Source: CAD feature listing. Evaluate the final solid. Frame: model axes, mm. Face numbers are marked on the shaded views. Coordinates: 2 decimals unless noted, no trailing zeros. Loops run counter-clockwise (first coordinate to the right, second up) from the corner with the lowest first, then second, coordinate; pieces in that order, holes last. Notation, with made-up numbers: M 0.5,-19 L 17.5,-19 A27 cw 17.5,1 Z; hole C 73.25,42 d7. An arc over 180 degrees is marked long. One line per question, with ' | ' between items. Start each with the question number.
1. Section query C-C, the plane x = 4. Output: boundary loops of the cut face in (y, z).
2. Pin query (flat end, axial travel): P1, Ø3, axis at x = 12.5, y = 0.5, coming from the +Z side; P2, Ø3, axis at x = 0, y = 0, coming from the -Z side; P3, Ø4, axis at x = -32.5, y = 0, coming from the -Z side; P4, Ø3, axis at x = -25, z = -17.5, coming from the +Y side. Return the tip coordinate at first contact, or that it passes through.
3. Section query A-A, the plane x = 25. Output: boundary loops of the cut face in (y, z).
4. Ray query, probe 1 along X at (y, z) = (-0.25, -13); probe 2 along Z at (x, y) = (25, -0.5); probe 3 along X at (y, z) = (-0.5, -17.5). Return the intervals inside material, ascending.
5. Section query B-B, the plane z = -17.5. Output: boundary loops of the cut face in (x, y), and give its area (3 significant figures).
6. Mould query, pull axis Z, two halves, no side actions, for the marked faces 1 and 2. Classes: pulls with the +Z half, pulls with the -Z half, needs draft (parallel to the pull), parting line crosses it, or undercut.
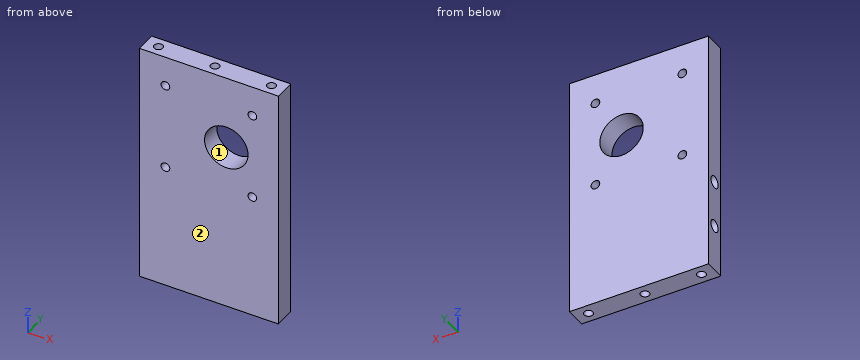
```python
from build123d import *

# Parameters (mm, degrees)
SKETCH1_W                  = 80
SKETCH1_H                  = 140
SKETCH1_R                  = 12.5
BOSS_EXTRUDE1_DEPTH        = 6
M6_TAPPED_HOLE1_D          = 5
M6_TAPPED_HOLE2_AT_2_COUNT = 2
M6_TAPPED_HOLE2_AT_2_PITCH = 32.5
M6_TAPPED_HOLE2_AT_3_COUNT = 2
M6_TAPPED_HOLE2_AT_3_PITCH = 65
M8X1_0_TAPPED_HOLE1_D      = 7
M8X1_0_TAPPED_HOLE1_DEPTH  = 19
M8X1_0_TAPPED_HOLE1_TIP    = 2.103012167


with BuildPart() as part:
    # Sketch1 → Boss-Extrude1 (new body, symmetric)
    with BuildSketch(Plane(origin=(0, 0, 0), x_dir=(1, 0, 0), z_dir=(0, 1, 0))):
        with Locations((0, 70)):
            Rectangle(SKETCH1_W, SKETCH1_H)
        with Locations((10, 42.5)):
            Circle(SKETCH1_R, mode=Mode.SUBTRACT)
    extrude(amount=BOSS_EXTRUDE1_DEPTH, both=True)

    # M6 Tapped Hole1 (through all)
    with Locations(Plane(origin=(0, 6, 0), x_dir=(1, 0, 0), z_dir=(0, 1, 0))):
        with Locations((-25, 67.5), (25, 67.5), (25, 17.5), (-25, 17.5)):
            Hole(M6_TAPPED_HOLE1_D / 2)

    # Sketch9 → M6 Tapped Hole2 (revolve, cut)
    with BuildSketch(Plane(origin=(32.5, 0, 0), x_dir=(0, -1, 0), z_dir=(1, 0, 0))):
        Polygon((0, 0), (0, 14.502151548), (2.5, 13), (2.5, 0), align=None)
    m6_tapped_hole2 = revolve(axis=Axis((32.5, 0, 6.35), (0, 0, -1)), mode=Mode.SUBTRACT)

    # M6 Tapped Hole2 at 2: M6 Tapped Hole2 ×2
    with Locations(*[(-i * M6_TAPPED_HOLE2_AT_2_PITCH, 0, 0) for i in range(1, M6_TAPPED_HOLE2_AT_2_COUNT)]):
        add(m6_tapped_hole2, mode=Mode.SUBTRACT)

    # M6 Tapped Hole2 at 3: M6 Tapped Hole2 ×2
    with Locations(*[(-i * M6_TAPPED_HOLE2_AT_3_PITCH, 0, 0) for i in range(1, M6_TAPPED_HOLE2_AT_3_COUNT)]):
        add(m6_tapped_hole2, mode=Mode.SUBTRACT)

    # Mirror1: M6 Tapped Hole2 across plane
    add(m6_tapped_hole2.mirror(Plane(origin=(0, 0, -70), x_dir=(1, 0, 0), z_dir=(0, 0, -1))), mode=Mode.SUBTRACT)

    # Mirror1 copy 1 sketch → Mirror1 copy 1 (revolve, cut)
    with BuildSketch(Plane(origin=(0, 0, -140), x_dir=(0, -1, 0), z_dir=(1, 0, 0))):
        Polygon((0, 0), (0, -14.502151548), (2.5, -13), (2.5, 0), align=None)
    revolve(axis=Axis((0, 0, -146.35), (0, 0, -1)), mode=Mode.SUBTRACT)

    # Mirror1 copy 2 sketch → Mirror1 copy 2 (revolve, cut)
    with BuildSketch(Plane(origin=(-32.5, 0, -140), x_dir=(0, -1, 0), z_dir=(1, 0, 0))):
        Polygon((0, 0), (0, -14.502151548), (2.5, -13), (2.5, 0), align=None)
    revolve(axis=Axis((-32.5, 0, -146.35), (0, 0, -1)), mode=Mode.SUBTRACT)

    # M8x1.0 Tapped Hole1
    with Locations(Plane.ZY.offset(40)):
        with Locations((-113, 0), (-86, 0)):
            Hole(M8X1_0_TAPPED_HOLE1_D / 2, depth=M8X1_0_TAPPED_HOLE1_DEPTH)
            with Locations((0, 0, -(M8X1_0_TAPPED_HOLE1_DEPTH + M8X1_0_TAPPED_HOLE1_TIP / 2))):  # 118° drill point
                Cone(0, M8X1_0_TAPPED_HOLE1_D / 2, M8X1_0_TAPPED_HOLE1_TIP, mode=Mode.SUBTRACT)


solid = part.part
```
Taken from the geometry:
1) outline: M -6,-140 L 6,-140 L 6,-53.47 L -6,-53.47 Z; M -6,-31.53 L 6,-31.53 L 6,0 L -6,0 Z
2) P1: z = 0 | P2: z = -126.4 | P3: z = -126.7 | P4: through
3) outline: M -6,-140 L 6,-140 L 6,-70 L -6,-70 Z; M -6,-65 L 6,-65 L 6,-20 L -6,-20 Z; M -6,-15 L 6,-15 L 6,0 L -6,0 Z
4) probe 1: -40 to -34.99, -30.01 to -2.49, 2.49 to 30.01, 34.99 to 40 | probe 2: -140 to -70, -65 to -20, -15 to 0 | probe 3: -40 to -27.5, -22.5 to 22.5, 27.5 to 40
5) outline: M -40,-6 L -27.5,-6 L -27.5,6 L -40,6 Z; M -22.5,-6 L 22.5,-6 L 22.5,6 L -22.5,6 Z; M 27.5,-6 L 40,-6 L 40,6 L 27.5,6 Z | area: 840 mm^2
6) face 1: undercut | face 2: needs draft
